For this review, take the finished solid that the model builds, in its own axes (mm). Face numbers are marked on the shaded views. A direction names the side the tool comes from. Round coordinates to 2 decimals unless told otherwise and drop trailing zeros. Loops run counter-clockwise (first coordinate to the right, second up) from the corner with the lowest first, then second, coordinate; pieces in that order, holes last.
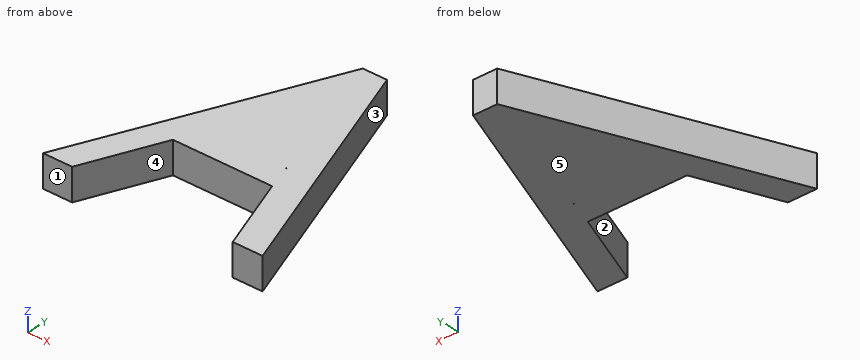
```python
from build123d import *

# Parameters (mm, degrees)
F1_DEPTH = 25.4
F2_DEPTH = 25.4


with BuildPart() as f1:
    # F0 (on Top) → F1 (new body)
    with BuildSketch(Plane.XY):
        Polygon((-123.5604166667, 188.4609023112), (-203.2, -13.8571532443), (-179.4756944444, -13.8571532443), (-154.6930555556, 50.2161106446), (-73.9510416667, 50.2161106446), (-48.8597222222, -13.8571532443), (-24.60625, -13.8571532443), (-103.8489583333, 188.4609023112), align=None)
        Polygon((-81.5007686615, 67.9640099406), (-152.8517007828, 67.9640099406), (-152.8517007828, 106.1364486814), (-139.8437470198, 106.1364486814), (-139.8437470198, 137.258246541), (-127.1816492081, 137.258246541), (-127.1816492081, 169.5059537888), (-101.4676243067, 169.5059537888), (-101.4676243067, 137.258246541), (-90.7859355211, 137.258246541), (-90.7859355211, 106.1364486814), (-81.5007686615, 106.1364486814), (-81.5007686615, 72.0230385523), (-81.2270833333, 71.2945828668), (-81.5007686615, 71.2945828668), align=None, mode=Mode.SUBTRACT)
    extrude(amount=F1_DEPTH)

    # F0 (on Top) → F2 (join)
    with BuildSketch(Plane.XY):
        Polygon((-146.4027777778, 71.2945828668), (-81.5007686615, 71.2945828668), (-81.5007686615, 72.0230385523), (-94.3173888512, 106.1364486814), (-133.1894430727, 106.1364486814), align=None)
        with BuildLine():
            Line((-122.7225694444, 133.7362495335), (-133.1894430727, 106.1364486814))
            Line((-133.1894430727, 106.1364486814), (-94.3173888512, 106.1364486814))
            Line((-94.3173888512, 106.1364486814), (-104.6868055556, 133.7362495335))
            add(Edge.make_bspline(
                [(-104.6868055556, 133.7362495335), (-105.3399663206, 135.4420771625), (-105.9985985773, 137.258246541)],
                knots=[0, 0, 0, 0.1438042201, 0.1438042201, 0.1438042201], degree=2))
            Line((-105.9985985773, 137.258246541), (-121.4879183379, 137.258246541))
            add(Edge.make_bspline(
                [(-121.4879183379, 137.258246541), (-122.0888459048, 135.5136460237), (-122.7225694444, 133.7362495335)],
                knots=[0.8877261445, 0.8877261445, 0.8877261445, 1, 1, 1], degree=2))
        make_face()
        with BuildLine():
            Line((-127.1816492081, 169.5059537888), (-127.1816492081, 137.258246541))
            Line((-127.1816492081, 137.258246541), (-121.4879183379, 137.258246541))
            add(Edge.make_bspline(
                [(-114.0354166667, 162.7963189779), (-116.7365084044, 151.0524418574), (-121.4879183379, 137.258246541)],
                knots=[0, 0, 0, 0.8877261445, 0.8877261445, 0.8877261445], degree=2))
            add(Edge.make_bspline(
                [(-105.9985985773, 137.258246541), (-109.9200284094, 148.071535305), (-114.0354166667, 162.7963189779)],
                knots=[0.1438042201, 0.1438042201, 0.1438042201, 1, 1, 1], degree=2))
            Line((-105.9985985773, 137.258246541), (-101.4676243067, 137.258246541))
            Line((-101.4676243067, 137.258246541), (-101.4676243067, 169.5059537888))
            Line((-101.4676243067, 169.5059537888), (-127.1816492081, 169.5059537888))
        make_face()
        with BuildLine():
            Line((-139.8437470198, 137.258246541), (-139.8437470198, 106.1364486814))
            Line((-139.8437470198, 106.1364486814), (-133.1894430727, 106.1364486814))
            Line((-133.1894430727, 106.1364486814), (-122.7225694444, 133.7362495335))
            add(Edge.make_bspline(
                [(-121.4879183379, 137.258246541), (-122.0888459048, 135.5136460237), (-122.7225694444, 133.7362495335)],
                knots=[0.8877261445, 0.8877261445, 0.8877261445, 1, 1, 1], degree=2))
            Line((-121.4879183379, 137.258246541), (-127.1816492081, 137.258246541))
            Line((-127.1816492081, 137.258246541), (-139.8437470198, 137.258246541))
        make_face()
        Polygon((-152.8517007828, 106.1364486814), (-152.8517007828, 67.9640099406), (-81.5007686615, 67.9640099406), (-81.5007686615, 71.2945828668), (-146.4027777778, 71.2945828668), (-133.1894430727, 106.1364486814), (-139.8437470198, 106.1364486814), align=None)
        with BuildLine():
            Line((-104.6868055556, 133.7362495335), (-94.3173888512, 106.1364486814))
            Line((-94.3173888512, 106.1364486814), (-90.7859355211, 106.1364486814))
            Line((-90.7859355211, 106.1364486814), (-90.7859355211, 137.258246541))
            Line((-90.7859355211, 137.258246541), (-101.4676243067, 137.258246541))
            Line((-101.4676243067, 137.258246541), (-105.9985985773, 137.258246541))
            add(Edge.make_bspline(
                [(-104.6868055556, 133.7362495335), (-105.3399663206, 135.4420771625), (-105.9985985773, 137.258246541)],
                knots=[0, 0, 0, 0.1438042201, 0.1438042201, 0.1438042201], degree=2))
        make_face()
        Polygon((-94.3173888512, 106.1364486814), (-81.5007686615, 72.0230385523), (-81.5007686615, 106.1364486814), (-90.7859355211, 106.1364486814), align=None)
        with BuildLine():
            add(Edge.make_bspline(
                [(-114.0354166667, 162.7963189779), (-116.7365084044, 151.0524418574), (-121.4879183379, 137.258246541)],
                knots=[0, 0, 0, 0.8877261445, 0.8877261445, 0.8877261445], degree=2))
            Line((-121.4879183379, 137.258246541), (-105.9985985773, 137.258246541))
            add(Edge.make_bspline(
                [(-105.9985985773, 137.258246541), (-109.9200284094, 148.071535305), (-114.0354166667, 162.7963189779)],
                knots=[0.1438042201, 0.1438042201, 0.1438042201, 1, 1, 1], degree=2))
        make_face()
    extrude(amount=F2_DEPTH)


solid = f1.part
```
(1) Insertion check: pin 1 Ø0.8 at (y, z) = (71.5, 18.5) entering from +X; pin 2 Ø1.5 at (y, z) = (88, 8) entering from -X; pin 3 Ø12 at (y, z) = (135, 9.5) entering from -X; pin 4 Ø10 at (x, y) = (-70.5, 127) entering from +Z. Each pin has a flat end and moves straight along its axis. Give the tip position at first contact, or say it passes through.
(2) For the marked faces 1 and 2, list the 3-axis set-ups (+Z, -Z, +X, -X, +Y, -Y) from which the entire face can be reached by the end or side of a thin tool; tool diameter is ignored.
(3) Add section D-D (x = -158). Give the boundary of the cut face in (y, z), plus the area to 3 significant figures.
(4) Add section C-C (y = 44). Give the boundary of the cut face in (x, z), plus the area to 3 significant figures.
(5) Add section A-A (z = 7). Give the boundary of the cut face in (x, y), plus the area to 3 significant figures.
(6) For L1, parallel to X at y = 22.5, z = 5; L2, parallel to X at y = -4, z = 10.75; L3, parallel to X at y = 78.5, z = 21.5, list the stretches that pass through material, from the lowest coordinate up.
(7) The part is to be moulded in two halves that separate along X. For the marked faces 3, 4 and 5, say which applies: pulls with the +X half, pulls with the -X half, needs draft (parallel to the pull), parting line crosses it, or undercut.
(8) Add section B-B (y = 4). Give the boundary of the cut face in (x, z), plus the area to 3 significant figures.
Outcome:
1. pin 1: stops at x = -57.88
1. pin 2: stops at x = -163.4
1. pin 3: stops at x = -146.97
1. pin 4: passes through
2. face 1: +Z, -Z, +X, -X, -Y
2. face 2: +Z, -Z, -Y
3. outline: (41.67, 0) - (100.97, 0) - (100.97, 25.4) - (41.67, 25.4) - close
3. area: 1,510 mm2
4. outline: (-180.43, 0) - (-157.1, 0) - (-157.1, 25.4) - (-180.43, 25.4) - close; (-71.52, 0) - (-47.27, 0) - (-47.27, 25.4) - (-71.52, 25.4) - close
4. area: 1,210 mm2
5. outline: (-203.2, -13.86) - (-179.48, -13.86) - (-154.69, 50.22) - (-73.95, 50.22) - (-48.86, -13.86) - (-24.61, -13.86) - (-103.85, 188.46) - (-123.56, 188.46) - close; hole (-81.5, 71.29) - (-81.23, 71.29) - (-81.5, 72.02) - close
5. area: 13,300 mm2
6. L1: x = -188.89 to -165.41, -63.1 to -38.85
6. L2: x = -199.32 to -175.66, -52.72 to -28.47
6. L3: x = -166.84 to -60.78
7. face 3: pulls with the +X half
7. face 4: undercut
7. face 5: needs draft
8. outline: (-196.17, 0) - (-172.57, 0) - (-172.57, 25.4) - (-196.17, 25.4) - close; (-55.85, 0) - (-31.6, 0) - (-31.6, 25.4) - (-55.85, 25.4) - close
8. area: 1,220 mm2
